Geometry check sheet. Reference: the model listing, model coordinates, mm. Round coordinates to 2 decimals unless told otherwise and drop trailing zeros. Order: outer loops, then holes, each group sorted by start corner. A loop starts at its lowest first (then second) coordinate and runs counter-clockwise, first axis right, second up.
(1) Cross-section at B-B on y = -1.5. Enter the section's corners in (x, z), and give its area (3 significant figures).
(2) Gauge pin test, flat end, axial feed: P1, Ø5, axis at y = -1, z = 2, coming from the +X side. Record the tip position at first contact, or that the pin passes through.
(3) Thickness scan on L1, parallel to Z at x = 1.5, y = 0; L2, parallel to Z at x = 1.4, y = 2.25; L3, parallel to Y at x = 0.85, z = -0.75. Record the ranges inside material, lowest first.
(4) Draft check along Y on faces 1 (the face through (1.04, 3.4, 2.52)), 2 (the face through (2.108, 3, 0)), 3 (the face through (1, -4.23, 0)), 4 (the face through (1.04, -0.54, 2.44)). Enter one of: pulls with the +Y half, pulls with the -Y half, needs draft (parallel to the pull), parting line crosses it, or undercut.
(5) Cross-section at C-C on x = 1.35. Enter the section's corners in (y, z).
(6) Cross-section at D-D on y = 3.5. Enter the section's corners in (x, z).
(7) Cross-section at A-A on z = 1.75. Enter the section's corners in (x, y), and give its area (3 significant figures).
Autodesk Inventor part; units mm, degrees
ref_plane "YZ Plane" through (0, 0, 0) normal (1, 0, 0) x (0, 1, 0)
ref_plane "XZ Plane" through (0, 0, 0) normal (0, 1, 0) x (-1, 0, 0)
ref_plane "XY Plane" through (0, 0, 0) normal (0, 0, 1) x (1, 0, 0)
sketch "Sketch1" plane through (0, 0, 0) normal (1, 0, 0) x (0, 1, 0)
  circle A0 centre (0, 0) radius 2.5
  line L0 (5.2285, 0) -> (1.6157, -4.9726)
  line L1 (1.6157, -4.9726) -> (-4.23, -3.0733)
  line L2 (-4.23, -3.0733) -> (-4.23, 3.0733)
  line L3 (-4.23, 3.0733) -> (1.6157, 4.9726)
  line L4 (1.6157, 4.9726) -> (5.2285, 0)
  dimension "d0" = 5
extrude "Extrusion1" add sketch "Sketch1" along normal blind 2.1082
properties part number "Bracket"
Found:
1. outline: (0, -3.96) - (2.11, -3.96) - (2.11, -2) - (0, -2) - close; (0, 2) - (2.11, 2) - (2.11, 3.96) - (0, 3.96) - close
1. area: 8.27 mm2
2. P1: stops at x = 2.11
3. L1: z = -4.45 to -2.5, 2.5 to 4.45
3. L2: z = -4.1 to -1.09, 1.09 to 4.1
3. L3: y = -4.23 to -2.38, 2.38 to 4.68
4. face 1: pulls with the +Y half
4. face 2: needs draft
4. face 3: pulls with the -Y half
4. face 4: undercut
5. outline: (-4.23, -3.07) - (1.62, -4.97) - (5.23, 0) - (1.62, 4.97) - (-4.23, 3.07) - close; hole circle Ø5 at (0, 0)
6. outline: (0, -2.38) - (2.11, -2.38) - (2.11, 2.38) - (0, 2.38) - close
7. outline: (0, -4.23) - (2.11, -4.23) - (2.11, -1.79) - (0, -1.79) - close; (0, 1.79) - (2.11, 1.79) - (2.11, 3.96) - (0, 3.96) - close
7. area: 9.73 mm2
